Could you check a few things on this model? Use its own coordinates, in mm. Face numbers are marked on the shaded views. A direction names the side the tool comes from. Round coordinates to 2 decimals unless told otherwise and drop trailing zeros. Loops run counter-clockwise (first coordinate to the right, second up) from the corner with the lowest first, then second, coordinate; pieces in that order, holes last. Notation, with made-up numbers: M 53.5,23 L 71.5,23 A28 cw 71.5,62 Z; hole C -2.75,85.25 d7. An arc over 180 degrees is marked long. One line per item, written item: value. Start each with the question number.
Q1. Imagine slicing it at B-B (y = 0). Please give me the cut outline in (x, z) (3 decimals).
Q2. Which directions (+Z, -Z, +X, -X, +Y, -Y) give clear straight access to the entire face, cutting with the end or side of a thin tool? Please do the marked faces 1, 2, 3 and 4.
Q3. Imagine slicing it at C-C (x = 0). Please give me the cut outline in (y, z) (3 decimals), then the cut area to 3 significant figures.
Q4. Imagine slicing it at D-D (x = -43). Please give me the cut outline in (y, z) (3 decimals), then the cut area to 3 significant figures.
Q5. Imagine slicing it at A-A (z = 0). Please give me the cut outline in (x, y) (3 decimals), then the cut area to 3 significant figures.
Q6. I'm going to push flat-ended pins straight in: pin 1 Ø10 at (y, z) = (-12, 8) entering from +X; pin 2 Ø4 at (x, z) = (48.5, 6) entering from +Y; pin 3 Ø5 at (x, y) = (46, 7.5) entering from -Z; pin 4 Ø6 at (x, y) = (52, 0.5) entering from -Z (3 decimals). Where does each tip first touch, or does it pass through?
Q7. Please list where these lines run through material, in increasing order: line 1 along X through (y, z) = (-4.5, 10.5); line 2 along Z through (x, y) = (-11.5, -1) (3 decimals); line 3 along X through (y, z) = (0, -46).
from build123d import *

# Parameters (mm, degrees)
F0_R     = 15.875
F1_DEPTH = 15.875
F2_R     = 6.35
F3_DEPTH = 44.45
F4_R     = 4.445
F5_DEPTH = 66.04


with BuildPart() as f1:
    # F0 (on Top) → F1 (new body, symmetric)
    with BuildSketch(Plane.XY):
        Circle(F0_R)
    extrude(amount=F1_DEPTH, both=True)

    # F2 (on face) → F3 (join)
    with BuildSketch(Plane(origin=(0, 0, -15.875), x_dir=(1, 0, 0), z_dir=(0, 0, -1))):
        Circle(F2_R)
    extrude(amount=F3_DEPTH)

    # F4 (on Right) → F5 (join, symmetric)
    with BuildSketch(Plane.YZ):
        Circle(F4_R)
    extrude(amount=F5_DEPTH, both=True)


solid = f1.part
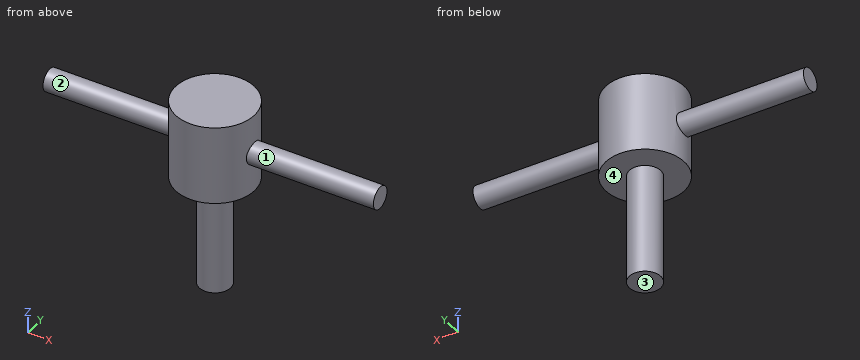
Report:
1. outline: M -66.04,-4.445 L -15.875,-4.445 L -15.875,-15.875 L -6.35,-15.875 L -6.35,-60.325 L 6.35,-60.325 L 6.35,-15.875 L 15.875,-15.875 L 15.875,-4.445 L 66.04,-4.445 L 66.04,4.445 L 15.875,4.445 L 15.875,15.875 L -15.875,15.875 L -15.875,4.445 L -66.04,4.445 Z
2. face 1: +X
2. face 2: -X
2. face 3: -Z, +X, -X, +Y, -Y
2. face 4: -Z
3. outline: M -15.875,-15.875 L -6.35,-15.875 L -6.35,-60.325 L 6.35,-60.325 L 6.35,-15.875 L 15.875,-15.875 L 15.875,15.875 L -15.875,15.875 Z
3. area: 1,570 mm²
4. outline: C 0,0 d8.89
4. area: 62.1 mm²
5. outline: M -66.04,-4.445 L -15.24,-4.445 A15.875 ccw 15.24,-4.445 L 66.04,-4.445 L 66.04,4.445 L 15.24,4.445 A15.875 ccw -15.24,4.445 L -66.04,4.445 Z
5. area: 1,690 mm²
6. pin 1: stops at x = 14.25
6. pin 2: stops at y = 1.94
6. pin 3: passes through
6. pin 4: stops at z = -4.445
7. line 1: x = -15.22 to 15.22
7. line 2: z = -15.875 to 15.875
7. line 3: x = -6.35 to 6.35
